```python
from build123d import *

# Parameters (mm, degrees)
EXTRUDE_1_DEPTH              = 5
EXTRUDE_1_DEPTH_BACK         = 2
FILLET_1_R                   = 10
EXTRUDE_2_DEPTH              = 2
SKETCH_7_R                   = 5
EXTRUDE_4_DEPTH              = 27
SKETCH_9_R                   = 29.5
CUT_EXTRUDE_2_DEPTH          = 199.967077983
SKETCH_6_R                   = 5
EXTRUDE_6_DEPTH              = 27
M4X0_5_1_D                   = 3.5
M4X0_5_1_DEPTH               = 9.5
M4X0_5_1_CSINK_D             = 4.05
M4X0_5_1_CSINK_ANGLE         = 90
M4X0_5_1_TIP                 = 1.051506083
SKETCH_12_R                  = 14
CUT_EXTRUDE_3_DEPTH          = 7
HOLE_WIZARD_M4_1_D           = 3.3
HOLE_WIZARD_M4_1_DEPTH       = 10.1
HOLE_WIZARD_M4_1_CSINK_D     = 4.05
HOLE_WIZARD_M4_1_CSINK_ANGLE = 90
HOLE_WIZARD_M4_1_TIP         = 0.991420021
PATTERN_CIRCULAR_1_COUNT     = 8


# Read off the part's stored shape, not the designer's step: M4 螺纹孔2
with BuildPart() as part:
    # 草图1 → 凸台-拉伸1 (new, two sides: drawn at the far end of the back side and taken through both)
    with BuildSketch(Plane(origin=(0, 0, 0), x_dir=(1, 0, 0), z_dir=(0, 1, 0)).offset(-EXTRUDE_1_DEPTH_BACK)):
        with BuildLine():
            Line((28.36210367, 15.823673932), (59.117479337, 105.823673932))
            ThreePointArc((59.117479337, 105.823673932), (0, 164.941153269), (-59.117479337, 105.823673932))
            Line((-59.117479337, 105.823673932), (-59.117478081, 105.811488283))
            Line((-59.117478081, 105.811488283), (-59.108203667, 15.82367441))
            Line((-59.108203667, 15.82367441), (11.786941507, -119.17632559))
            Line((11.786941507, -119.17632559), (2.233923801, -164.17632559))
            ThreePointArc((2.233923801, -164.17632559), (14.171961552, -186.818592843), (38.601140216, -179.176326068))
            Line((38.601140216, -179.176326068), (58.357719046, -109.176326068))
            Line((58.357719046, -109.176326068), (28.36210367, 15.823673932))
        make_face()
    extrude(amount=EXTRUDE_1_DEPTH + EXTRUDE_1_DEPTH_BACK)

    # 圆角1
    fillet_1_edges = [part.edges().sort_by_distance(p)[0] for p in [
        (11.786941507, 1.5, 119.17632559),
        (-59.108203667, 1.5, -15.82367441),
        (59.117479337, 1.5, -105.823673932),
        (28.36210367, 1.5, -15.823673932),
        (58.357719046, 1.5, 109.176326068),
        (38.601140216, 1.5, 179.176326068),
    ]]
    fillet(fillet_1_edges, radius=FILLET_1_R)

    # 草图8 → 凸台-拉伸2 (add)
    with BuildSketch(Plane(origin=(0, 5, 0), x_dir=(1, 0, 0), z_dir=(0, 1, 0))):
        with BuildLine():
            Line((29.300361737, 18.569315114), (58.554588826, 104.176477469))
            ThreePointArc((58.554588826, 104.176477469), (58.98180751, 105.930695077), (59.086633883, 107.733139709))
            ThreePointArc((59.086633883, 107.733139709), (-0.95485745, 164.933441402), (-59.117479337, 105.823673932))
            Line((-59.117479337, 105.823673932), (-59.108457771, 18.289190078))
            ThreePointArc((-59.108457771, 18.289190078), (-58.817462925, 15.895388783), (-57.961893059, 13.640846069))
            Line((-57.961893059, 13.640846069), (10.108867752, -115.980902881))
            ThreePointArc((10.108867752, -115.980902881), (11.161474402, -119.262675904), (11.037439917, -122.706892851))
            Line((11.037439917, -122.706892851), (2.233923801, -164.17632559))
            ThreePointArc((2.233923801, -164.17632559), (13.031285464, -186.305812614), (37.116640576, -181.187914225))
            ThreePointArc((37.116640576, -181.187914225), (38.296139318, -179.43577869), (39.081319631, -177.47499107))
            Line((39.081319631, -177.47499107), (57.648798745, -111.688118295))
            ThreePointArc((57.648798745, -111.688118295), (58.022811544, -109.169699075), (57.748719119, -106.63845545))
            Line((57.748719119, -106.63845545), (29.039148609, 13.002240988))
            ThreePointArc((29.039148609, 13.002240988), (28.774088822, 15.804343144), (29.300361737, 18.569315114))
        make_face()
    extrude(amount=EXTRUDE_2_DEPTH)

    # 草图7 → 凸台-拉伸4 (add)
    with BuildSketch(Plane(origin=(0, 5, 0), x_dir=(1, 0, 0), z_dir=(0, 1, 0))):
        with Locations(Location((0, -10.167611435, 0), (0, 0, 270))):
            Circle(SKETCH_7_R)
        with Locations(Location((10.962320581, -43.406557379, 0), (0, 0, 270))):
            Circle(SKETCH_7_R)
        with Locations(Location((21.924641163, -76.645503323, 0), (0, 0, 270))):
            Circle(SKETCH_7_R)
        with Locations(Location((32.886961744, -109.884449267, 0), (0, 0, 270))):
            Circle(SKETCH_7_R)
        with Locations(Location((27.862861404, -133.987984293, 0), (0, 0, 270))):
            Circle(SKETCH_7_R)
    extrude(amount=EXTRUDE_4_DEPTH)

    # 草图9 → 切除-拉伸2 (cut, through all)
    with BuildSketch(Plane(origin=(0, 7, 0), x_dir=(1, 0, 0), z_dir=(0, 1, 0))):
        with Locations(Location((0, 105.823673932, 0), (0, 0, 270))):
            Circle(SKETCH_9_R)
    extrude(amount=-CUT_EXTRUDE_2_DEPTH, mode=Mode.SUBTRACT)

    # 草图6 → 凸台-拉伸6 (add)
    with BuildSketch(Plane(origin=(0, 5, 0), x_dir=(1, 0, 0), z_dir=(0, 1, 0))):
        with Locations(Location((0, 155.823673932, 0), (0, 0, 270))):
            Circle(SKETCH_6_R)
        with Locations(Location((0, 55.823673932, 0), (0, 0, 270))):
            Circle(SKETCH_6_R)
        with Locations(Location((-50, 105.823673932, 0), (0, 0, 270))):
            Circle(SKETCH_6_R)
        with Locations(Location((-39.108203667, 15.82367441, 0), (0, 0, 270))):
            Circle(SKETCH_6_R)
    extrude(amount=EXTRUDE_6_DEPTH)

    # M4x0.5 螺纹孔1
    with Locations(Plane(origin=(0, 32, 0), x_dir=(1, 0, 0), z_dir=(0, 1, 0))):
        with Locations((0, 155.823673932), (-50, 105.823673932), (0, 55.823673932), (-39.108203667, 15.82367441), (0, -10.167611435), (10.962320581, -43.406557379), (21.924641163, -76.645503323), (32.886961744, -109.884449267), (27.862861404, -133.987984293)):
            CounterSinkHole(M4X0_5_1_D / 2, M4X0_5_1_CSINK_D / 2, depth=M4X0_5_1_DEPTH, counter_sink_angle=M4X0_5_1_CSINK_ANGLE)
            with Locations((0, 0, -(M4X0_5_1_DEPTH + M4X0_5_1_TIP / 2))):  # 118° drill point
                Cone(0, M4X0_5_1_D / 2, M4X0_5_1_TIP, mode=Mode.SUBTRACT)

    # 草图12 → 切除-拉伸3 (cut)
    with BuildSketch(Plane(origin=(0, 7, 0), x_dir=(1, 0, 0), z_dir=(0, 1, 0))):
        with Locations(Location((21.7979386, -168.329556252, 0), (0, 0, 270))):
            Circle(SKETCH_12_R)
    extrude(amount=-CUT_EXTRUDE_3_DEPTH, mode=Mode.SUBTRACT)

    # M4 螺纹孔1
    with Locations(Plane(origin=(0, -2, 0), x_dir=(-1, 0, 0), z_dir=(0, -1, 0))):
        with Locations((-21.7979386, -168.329556252)):
            CounterSinkHole(HOLE_WIZARD_M4_1_D / 2, HOLE_WIZARD_M4_1_CSINK_D / 2, depth=HOLE_WIZARD_M4_1_DEPTH, counter_sink_angle=HOLE_WIZARD_M4_1_CSINK_ANGLE)
            with Locations((0, 0, -(HOLE_WIZARD_M4_1_DEPTH + HOLE_WIZARD_M4_1_TIP / 2))):  # 118° drill point
                Cone(0, HOLE_WIZARD_M4_1_D / 2, HOLE_WIZARD_M4_1_TIP, mode=Mode.SUBTRACT)

    # M4 螺纹孔2 outline → M4 螺纹孔2 (revolve, cut)
    with BuildSketch(Plane.XY.offset(-148.323673932)):
        Polygon((1.65, -1.625), (1.65, 7), (0, 7), (0, -2), (2.025, -2), align=None)
    hole_wizard_m4_2 = revolve(axis=Axis((0, 0, -148.323673932), (0, 1, 0)), mode=Mode.SUBTRACT)

    # 阵列(圆周)1: M4 螺纹孔2 ×8 about axis
    pattern_circular_1_axis = Axis((0, 0, -105.823673932), (0, 1, 0))
    for i in range(1, PATTERN_CIRCULAR_1_COUNT):
        add(hole_wizard_m4_2.rotate(pattern_circular_1_axis, i * 360 / PATTERN_CIRCULAR_1_COUNT), mode=Mode.SUBTRACT)


solid = part.part
```
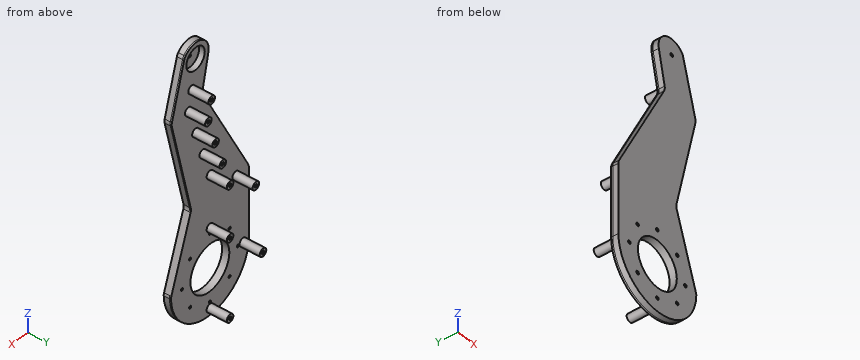
Geometry: final body of the model. Coordinates: model frame, mm. Give positions to 0.01 mm unless a question says otherwise; leave off trailing zeros. Loops run counter-clockwise (first coordinate to the right, second up) from the corner with the lowest first, then second, coordinate; pieces in that order, holes last. Notation, with made-up numbers: (-0.75, 84.5) -> (16.25, 84.5) arc R7 cw to (16.25, 89.5) -> close; hole circle Ø10 at (26.5, -22.75). An arc over 180 degrees is marked (long way). Use CSV: the item, a comma, the result in double quotes.
(1) Cut plane A-A (y = 27.5). Count the separate pieces of the cut face and the enclosed holes in it, plus the area to 3 significant figures.
From the geometry:
separate pieces,"9"
enclosed holes,"9"
area,"620 mm^2"
(2) First-contact query: P1, Ø4.5, axis at x = -39.11, z = -15.82, coming from the +Y side; P2, Ø10, axis at x = 19, y = 24, coming from the -Z side; P3, Ø5, axis at x = -22, z = -34, coming from the +Y side; P4, Ø12, axis at x = -43.5, y = 6.5, coming from the -Z side. Flat tips, straight axial feed; report the tip coordinate or a pass-through.
From the geometry:
P1,"y = 32"
P2,"z = 39.44"
P3,"y = 7"
P4,"z = -151.53"
(3) Cut plane B-B (x = -22.5). Output: boundary loops of the cut face in (y, z).
From the geometry:
outline,"(-2, -160.49) -> (7, -160.49) -> (7, -124.9) -> (-2, -124.9) -> close; (-2, -86.74) -> (7, -86.74) -> (7, 53.89) -> (-2, 53.89) -> close"
(4) Cut plane C-C (z = -129). Output: boundary loops of the cut face in (x, y).
From the geometry:
outline,"(-54.39, -2) -> (-18.25, -2) -> (-18.25, 7) -> (-54.39, 7) -> close; (18.25, -2) -> (54.39, -2) -> (54.39, 7) -> (18.25, 7) -> close"
(5) Cut plane D-D (z = -31). Output: boundary loops of the cut face in (x, y), plus the area to 3 significant figures.
From the geometry:
outline,"(-59.11, -2) -> (33.55, -2) -> (33.55, 7) -> (-59.11, 7) -> close"
area,"834 mm^2"
(6) Ray query, line 1 along Z through (x, y) = (1, 14.5); line 2 along Y through (x, z) = (35.5, 42); line 3 along X through (y, z) = (6, -119.5). Return the intervals inside material, ascending. Write a range as [from, to].
From the geometry:
line 1,"[-160.72, -150.92], [-60.72, -50.92], [5.27, 15.07]"
line 2,"[-2, 7]"
line 3,"[-57.51, -26.14], [26.14, 57.51]"
